from build123d import *

# Parameters (mm, degrees)
SKETCH3_W           = 40
SKETCH3_H           = 80
BOSS_EXTRUDE1_DEPTH = 10
SKETCH4_R           = 10
CUT_EXTRUDE4_DEPTH  = 7
BOSS_EXTRUDE3_DEPTH = 40
CUT_EXTRUDE5_DEPTH  = 40


with BuildPart() as part:
    # Sketch3 → Boss-Extrude1 (new body)
    with BuildSketch(Plane.XY):
        Rectangle(SKETCH3_W, SKETCH3_H)
    extrude(amount=BOSS_EXTRUDE1_DEPTH)

    # Sketch4 → Cut-Extrude4 (cut)
    with BuildSketch(Plane.XY.offset(10)):
        with Locations((0, 25)):
            Circle(SKETCH4_R)
        Circle(SKETCH4_R)
        with Locations((0, -25)):
            Circle(SKETCH4_R)
    extrude(amount=-CUT_EXTRUDE4_DEPTH, mode=Mode.SUBTRACT)

    # Sketch5 → Revolve1 (revolve)
    with BuildSketch(Plane.XY.offset(10)):
        with BuildLine():
            Line((16, 38.5), (16, 33.5))
            ThreePointArc((16, 33.5), (13.5, 36), (16, 38.5))
        make_face()
    revolve(axis=Axis((16, 38.5, 10), (0, -1, 0)))

    # Sketch7 → Revolve2 (revolve)
    with BuildSketch(Plane.XY.offset(10)):
        with BuildLine():
            Line((-16, -33.5), (-16, -38.5))
            ThreePointArc((-16, -38.5), (-18.5, -36), (-16, -33.5))
        make_face()
        with BuildLine():
            Line((-16, 38.5), (-16, 33.5))
            ThreePointArc((-16, 33.5), (-18.5, 36), (-16, 38.5))
        make_face()
    revolve(axis=Axis((-16, -33.5, 10), (0, -1, 0)))

    # Sketch8 → Revolve3 (revolve)
    with BuildSketch(Plane.XY.offset(10)):
        with BuildLine():
            Line((16, -33.5), (16, -38.5))
            ThreePointArc((16, -38.5), (13.5, -36), (16, -33.5))
        make_face()
    revolve(axis=Axis((16, -33.5, 10), (0, -1, 0)))

    # Sketch12 → Boss-Extrude3 (add)
    with BuildSketch(Plane.ZY.offset(20)):
        with BuildLine():
            Line((0, 10), (0, -10))
            ThreePointArc((0, -10), (-10, 0), (0, 10))
        make_face()
    extrude(amount=-BOSS_EXTRUDE3_DEPTH)

    # Sketch13 → Cut-Extrude5 (cut)
    with BuildSketch(Plane.ZY.offset(20)):
        with BuildLine():
            Line((0, 5), (0, -5))
            ThreePointArc((0, -5), (-5, 0), (0, 5))
        make_face()
    extrude(amount=-CUT_EXTRUDE5_DEPTH, mode=Mode.SUBTRACT)


solid = part.part
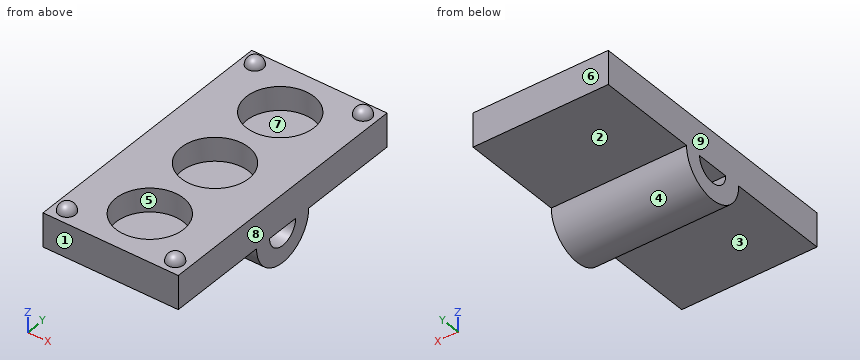
Here's how the part is built. I have some questions about the finished solid (model axes, mm). Face numbers are marked on the shaded views. A direction names the side the tool comes from. Round coordinates to 2 decimals unless told otherwise and drop trailing zeros. Order: outer loops, then holes, each group sorted by start corner. A loop starts at its lowest first (then second) coordinate and runs counter-clockwise, first axis right, second up. Notation, with made-up numbers: (86, 14) -> (91, 14) arc R20 cw to (91, 38) -> close; hole circle Ø6 at (-21.5, 87.5). An arc over 180 degrees is marked (long way). Use CSV: the item, a comma, the result in double quotes.
1. Which directions (+Z, -Z, +X, -X, +Y, -Y) give clear straight access to the entire face, cutting with the end or side of a thin tool? Please do the marked faces 1, 2, 3, 4 and 5.
Recorded:
face 1,"+Z, -Z, +X, -X, -Y"
face 2,"-Z, +X, -X, +Y"
face 3,"-Z, +X, -X, -Y"
face 4,"-Z, +X, -X"
face 5,"+Z"
2. I'm going to push flat-ended pins straight in: P1, Ø22, axis at x = 4.5, y = 28, coming from the +Z side; P2, Ø16, axis at x = 0, y = 25, coming from the +Z side; P3, Ø1, axis at y = -28, z = -1, coming from the -X side; P4, Ø9, axis at x = 3, y = 24, coming from the -Z side. Where does each tip first touch, or does it pass through?
Recorded:
P1,"stops at z = 10"
P2,"stops at z = 3"
P3,"passes through"
P4,"stops at z = 0"
3. I want a section at D-D on y = -19. List the corners of the cut face in (x, z) for me.
Recorded:
outline,"(-20, 0) -> (20, 0) -> (20, 10) -> (8, 10) -> (8, 3) -> (-8, 3) -> (-8, 10) -> (-20, 10) -> close"
4. I want a section at C-C on z = 5.25. List the corners of the cut face in (x, y) for me.
Recorded:
outline,"(-20, -40) -> (20, -40) -> (20, 40) -> (-20, 40) -> close; hole circle Ø20 at (0, -25); hole circle Ø20 at (0, 0); hole circle Ø20 at (0, 25)"
5. I want a section at B-B on x = 0. List the corners of the cut face in (y, z) for me.
Recorded:
outline,"(-40, 0) -> (-10, 0) arc R10 ccw to (10, 0) -> (40, 0) -> (40, 10) -> (35, 10) -> (35, 3) -> (15, 3) -> (15, 10) -> (10, 10) -> (10, 3) -> (-10, 3) -> (-10, 10) -> (-15, 10) -> (-15, 3) -> (-35, 3) -> (-35, 10) -> (-40, 10) -> close; hole (-5, 0) arc R5 ccw to (5, 0) -> close"
6. Thinking about a two-plate mould opening in X: for the marked faces 6, 7, 8 and 9, which applies, pulls with the +X half, pulls with the -X half, needs draft (parallel to the pull), parting line crosses it, or undercut?
Recorded:
face 6,"needs draft"
face 7,"undercut"
face 8,"pulls with the +X half"
face 9,"pulls with the -X half"
7. I need wall thicknesses on line 1 along Y through (x, z) = (0, 4.5); line 2 along Z through (x, y) = (8, -24.5); line 3 along Y through (x, z) = (0.5, -2). Which ranges of each line are inside material? Lowest first, please.
Recorded:
line 1,"y = -40 to -35, -15 to -10, 10 to 15, 35 to 40"
line 2,"z = 0 to 3"
line 3,"y = -9.8 to -4.58, 4.58 to 9.8"
8. I want a section at A-A on y = 0. List the corners of the cut face in (x, z) for me.
Recorded:
outline,"(-20, -10) -> (20, -10) -> (20, -5) -> (-20, -5) -> close; (-20, 0) -> (20, 0) -> (20, 10) -> (10, 10) -> (10, 3) -> (-10, 3) -> (-10, 10) -> (-20, 10) -> close"
